Check sheet for the modelled part. Datum: model origin and axes. Units: mm. A direction names the side the tool comes from. Coordinates: 2 decimals unless noted, no trailing zeros. Order: outer loops, then holes, each group sorted by start corner. A loop starts at its lowest first (then second) coordinate and runs counter-clockwise, first axis right, second up.
Autodesk Inventor part; units mm, degrees
ref_plane "YZ Plane" through (0, 0, 0) normal (1, 0, 0) x (0, 1, 0)
ref_plane "XZ Plane" through (0, 0, 0) normal (0, 1, 0) x (-1, 0, 0)
ref_plane "XY Plane" through (0, 0, 0) normal (0, 0, 1) x (1, 0, 0)
sketch "Sketch1" plane through (0, 0, 0) normal (0, 0, 1) x (1, 0, 0)
  line L0 (0, 0) -> (50.8, 0)
  line L1 (50.8, 0) -> (50.8, 25.4)
  line L2 (50.8, 25.4) -> (0, 25.4)
  line L3 (0, 25.4) -> (0, 0)
  dimension "d0" = 25.4
  dimension "d1" = 50.8
extrude "Extrusion1" add sketch "Sketch1" along normal blind 635
shell "Shell1" thickness 3.175 removed faces 2 at (16.9333, 16.9333, 0) at (33.8667, 8.4667, 635)
sketch "Sketch2" plane through (0, 25.4, 0) normal (0, 1, 0) x (1, 0, 0)
  line L0 (0, -635) -> (50.8, -635)
  line L1 (50.8, 0) -> (0, 0)
  line L2 (0, 0) -> (0, -635)
  line L3 (12.7, 0) -> (12.7, -50.8) construction
  line L4 (12.7, -50.8) -> (12.7, -101.6) construction
  line L5 (12.7, -101.6) -> (12.7, -533.4) construction
  line L6 (12.7, -533.4) -> (12.7, -584.2) construction
  line L7 (12.7, -584.2) -> (12.7, -635) construction
  circle A0 centre (12.7, -50.8) radius 3.175
  circle A1 centre (12.7, -101.6) radius 3.175
  circle A2 centre (12.7, -533.4) radius 3.175
  circle A3 centre (12.7, -584.2) radius 3.175
  dimension "d4" = 12.7
  dimension "d5" = 50.8
  dimension "d6" = 50.8
  dimension "d7" = 6.35
  dimension "d8" = 6.35
  dimension "d9" = 6.35
  dimension "d10" = 6.35
extrude "Extrusion2" cut sketch "Sketch2" against normal through all
sketch "Sketch3" plane through (0, 25.4, 0) normal (0, 1, 0) x (1, 0, 0)
  line L0 (50.8, 0) -> (0, 0)
  line L1 (0, 0) -> (0, -635)
  line L2 (12.7, 0) -> (12.7, -127) construction
  line L3 (12.7, -127) -> (12.7, -152.4) construction
  line L4 (12.7, -152.4) -> (12.7, -177.8) construction
  line L5 (12.7, -177.8) -> (12.7, -203.2) construction
  line L6 (12.7, -203.2) -> (12.7, -228.6) construction
  line L7 (12.7, -228.6) -> (12.7, -254) construction
  line L8 (12.7, -254) -> (12.7, -279.4) construction
  line L9 (12.7, -279.4) -> (12.7, -304.8) construction
  line L10 (12.7, -304.8) -> (12.7, -330.2) construction
  line L11 (12.7, -330.2) -> (12.7, -355.6) construction
  line L12 (12.7, -355.6) -> (12.7, -381) construction
  line L13 (12.7, -381) -> (12.7, -406.4) construction
  line L14 (12.7, -406.4) -> (12.7, -431.8) construction
  line L15 (12.7, -431.8) -> (12.7, -457.2) construction
  line L16 (12.7, -457.2) -> (12.7, -482.6) construction
  circle A0 centre (12.7, -457.2) radius 2.3813
  circle A1 centre (12.7, -431.8) radius 2.3813
  circle A2 centre (12.7, -406.4) radius 2.3813
  circle A3 centre (12.7, -381) radius 2.3813
  circle A4 centre (12.7, -355.6) radius 2.3813
  circle A5 centre (12.7, -330.2) radius 2.3813
  circle A6 centre (12.7, -304.8) radius 2.3813
  circle A7 centre (12.7, -279.4) radius 2.3813
  circle A8 centre (12.7, -254) radius 2.3813
  circle A9 centre (12.7, -228.6) radius 2.3813
  circle A10 centre (12.7, -203.2) radius 2.3813
  circle A11 centre (12.7, -177.8) radius 2.3813
  circle A12 centre (12.7, -152.4) radius 2.3813
  circle A13 centre (12.7, -127) radius 2.3813
  line L17 (12.7, -482.6) -> (12.7, -508) construction
  circle A14 centre (12.7, -482.6) radius 2.3813
  circle A15 centre (12.7, -510.4986) radius 2.3813
  dimension "d14" = 12.7
  dimension "d15" = 25.4
  dimension "d16" = 127
  dimension "d17" = 4.7625
extrude "Extrusion3" cut sketch "Sketch3" against normal through all
properties part number "Frame_SideRail_Inner_2x1" material "Aluminum-6061"
(1) Cross-section at B-B (y = 9.75). Enter the section's corners in (x, z) (3 decimals).
Filled in:
outline: (0, 0) - (3.175, 0) - (3.175, 635) - (0, 635) - close; (47.625, 0) - (50.8, 0) - (50.8, 635) - (47.625, 635) - close
(2) Release check for a two-part mould opening along X. For faces 3 (the flat face through (25, 23, 0)), 4 (the flat face through (0, 13, 313)), 5 (the flat face through (26, 22.225, 313)) record: +X half, -X half, draft (parallel to the pull), parting line (faces both ways), or undercut.
Filled in:
face 3: draft
face 4: -X half
face 5: undercut
(3) Cross-section at A-A (x = 31.5). Enter the section's corners in (y, z) (3 decimals), and give its area (3 significant figures).
Filled in:
outline: (0, 0) - (3.175, 0) - (3.175, 635) - (0, 635) - close; (22.225, 0) - (25.4, 0) - (25.4, 635) - (22.225, 635) - close
area: 4,030 mm2
(4) Tool access check on faces 1 (the flat face through (47.625, 13, 313)), 2 (the flat face through (25, 23, 635)). Record the directions out of +Z, -Z, +X, -X, +Y, -Y that give a thin tool (end or side, any length) a straight path to the whole face; none if there is none.
Filled in:
face 1: +Z, -Z
face 2: +Z, +X, -X, +Y, -Y
(5) Cross-section at C-C (z = 41). Enter the section's corners in (x, y) (3 decimals).
Filled in:
outline: (0, 0) - (50.8, 0) - (50.8, 25.4) - (0, 25.4) - close; hole (3.175, 3.175) - (47.625, 3.175) - (47.625, 22.225) - (3.175, 22.225) - close
(6) Thickness scan on probe 1 along X at (y, z) = (4, 329.5) (3 decimals); probe 2 along Y at (x, z) = (18, 328.5) (3 decimals); probe 3 along X at (y, z) = (1.95, 279.4). Record the ranges inside material, lowest first.
Filled in:
probe 1: x = 0 to 3.175, 47.625 to 50.8
probe 2: y = 0 to 3.175, 22.225 to 25.4
probe 3: x = 0 to 10.32, 15.08 to 50.8
(7) Go/stop test with a flat-tipped pin: P1, Ø10, axis at x = 41.5, y = 12, coming from the -Z side. Record where the tip stops, or that it passes through.
Filled in:
P1: passes through
